The model under review builds one solid part; all positions refer to its coordinate system, in mm. Coordinates: 2 decimals unless noted, no trailing zeros. Order: outer loops, then holes, each group sorted by start corner. A loop starts at its lowest first (then second) coordinate and runs counter-clockwise, first axis right, second up. Notation, with made-up numbers: M 66.5,54.25 L 125.5,54.25 A10 cw 125.5,70.25 Z; hole C 14.25,53 d9. An arc over 180 degrees is marked long. Answer in a Markdown table with one row per item.
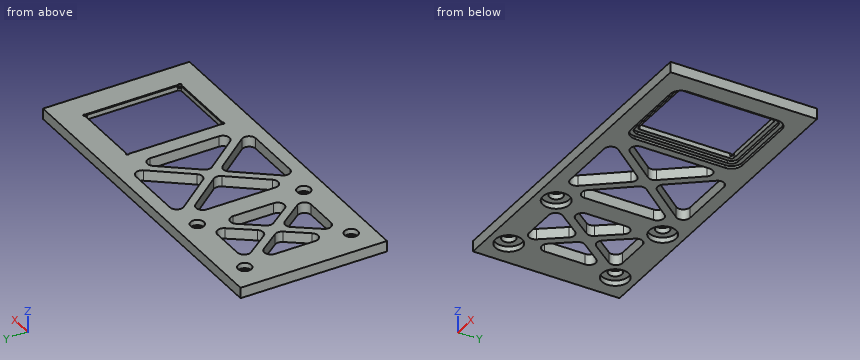
from build123d import *

# Parameters (mm, degrees)
SKETCH1_W           = 125
SKETCH1_H           = 55
SKETCH1_R           = 2.5
SKETCH1_W_2         = 27.05
SKETCH1_H_2         = 35.85
BOSS_EXTRUDE1_DEPTH = 4
SKETCH2_R           = 0.5
CUT_EXTRUDE1_DEPTH  = 1
FILLET1_R           = 1
FILLET2_R           = 1
SKETCH7_W           = 27.45
SKETCH7_H           = 36.25
CUT_EXTRUDE2_DEPTH  = 0.2
CUT_EXTRUDE3_DEPTH  = 2
CUT_EXTRUDE4_DEPTH  = 1
CUT_EXTRUDE5_DEPTH  = 137.623570441
CUT_EXTRUDE6_DEPTH  = 137.623570441
FILLET3_R           = 2.5
SKETCH12_R          = 5
CUT_EXTRUDE7_DEPTH  = 2


with BuildPart() as part:
    # Sketch1 → Boss-Extrude1 (new body)
    with BuildSketch(Plane.XY):
        with Locations((62.5, 27.5)):
            Rectangle(SKETCH1_W, SKETCH1_H)
        with Locations((10, 47.5)):
            Circle(SKETCH1_R, mode=Mode.SUBTRACT)
        with Locations((40, 47.5)):
            Circle(SKETCH1_R, mode=Mode.SUBTRACT)
        with Locations((10, 7.5)):
            Circle(SKETCH1_R, mode=Mode.SUBTRACT)
        with Locations((40, 7.5)):
            Circle(SKETCH1_R, mode=Mode.SUBTRACT)
        with Locations((101.25, 27.5)):
            Rectangle(SKETCH1_W_2, SKETCH1_H_2, mode=Mode.SUBTRACT)
    extrude(amount=BOSS_EXTRUDE1_DEPTH)

    # Sketch2 → Cut-Extrude1 (cut)
    with BuildSketch(Plane.XY.offset(4)):
        with Locations((87.725, 45.425)):
            Circle(SKETCH2_R)
        with Locations((114.775, 45.425)):
            Circle(SKETCH2_R)
        with Locations((87.725, 9.575)):
            Circle(SKETCH2_R)
        with Locations((114.775, 9.575)):
            Circle(SKETCH2_R)
    extrude(amount=-CUT_EXTRUDE1_DEPTH, mode=Mode.SUBTRACT)

    # Fillet1
    # the kernel refuses this fillet: 1 mm, written as the material it adds along each edge
    with BuildSketch(Plane(origin=(114.775, 9.575, 0), x_dir=(-1, 0, 0), z_dir=(0, 0, 1))) as fillet1_piece_1_section:
        with BuildLine():
            CenterArc((FILLET1_R, -FILLET1_R), FILLET1_R, 90, 90)
            Line((0, -FILLET1_R), (0, 0))
            Line((0, 0), (FILLET1_R, 0))
        make_face()
    fillet1_piece_1 = extrude(amount=5.5, mode=Mode.PRIVATE)
    fillet1_piece_1 = split(fillet1_piece_1, bisect_by=Plane(origin=(114.157064257, 9.617383677, 4), z_dir=(0, 0, -1)), keep=Keep.TOP, mode=Mode.PRIVATE)
    fillet1_piece_1 = fillet1_piece_1 - Plane(origin=(114.775, 9.575, 1.5), x_dir=(1, 0, 0), z_dir=(0, 0, 1)) * Cylinder(0.5, 16, mode=Mode.PRIVATE)
    add(fillet1_piece_1)
    with BuildSketch(Plane(origin=(114.775, 9.575, 0), x_dir=(-1, 0, 0), z_dir=(0, 0, 1)), Plane(origin=(87.725, 9.575, 0), x_dir=(0, 1, 0), z_dir=(0, 0, 1)), Plane(origin=(114.775, 45.425, 0), x_dir=(0, -1, 0), z_dir=(0, 0, 1))) as fillet1_piece_2:
        with BuildLine():
            CenterArc((FILLET1_R, -FILLET1_R), FILLET1_R, 90, 90)
            Line((0, -FILLET1_R), (0, 0))
            Line((0, 0), (FILLET1_R, 0))
        make_face()
    extrude(amount=3)
    with BuildSketch(Plane(origin=(87.725, 9.575, 0), x_dir=(0, 1, 0), z_dir=(0, 0, 1))) as fillet1_piece_3_section:
        with BuildLine():
            CenterArc((FILLET1_R, -FILLET1_R), FILLET1_R, 90, 90)
            Line((0, -FILLET1_R), (0, 0))
            Line((0, 0), (FILLET1_R, 0))
        make_face()
    fillet1_piece_3 = extrude(amount=5.5, mode=Mode.PRIVATE)
    fillet1_piece_3 = split(fillet1_piece_3, bisect_by=Plane(origin=(87.767383677, 10.192935743, 4), z_dir=(0, 0, -1)), keep=Keep.TOP, mode=Mode.PRIVATE)
    fillet1_piece_3 = fillet1_piece_3 - Plane(origin=(87.725, 9.575, 1.5), x_dir=(1, 0, 0), z_dir=(0, 0, 1)) * Cylinder(0.5, 15, mode=Mode.PRIVATE)
    add(fillet1_piece_3)
    with BuildSketch(Plane(origin=(114.775, 45.425, 0), x_dir=(0, -1, 0), z_dir=(0, 0, 1))) as fillet1_piece_4_section:
        with BuildLine():
            CenterArc((FILLET1_R, -FILLET1_R), FILLET1_R, 90, 90)
            Line((0, -FILLET1_R), (0, 0))
            Line((0, 0), (FILLET1_R, 0))
        make_face()
    fillet1_piece_4 = extrude(amount=5.5, mode=Mode.PRIVATE)
    fillet1_piece_4 = split(fillet1_piece_4, bisect_by=Plane(origin=(114.732616323, 44.807064257, 4), z_dir=(0, 0, -1)), keep=Keep.TOP, mode=Mode.PRIVATE)
    fillet1_piece_4 = fillet1_piece_4 - Plane(origin=(114.775, 45.425, 1.5), x_dir=(1, 0, 0), z_dir=(0, 0, 1)) * Cylinder(0.5, 15, mode=Mode.PRIVATE)
    add(fillet1_piece_4)
    with BuildSketch(Plane(origin=(87.725, 45.425, 0), x_dir=(0, -1, 0), z_dir=(0, 0, 1))) as fillet1_piece_5_section:
        with BuildLine():
            CenterArc((FILLET1_R, FILLET1_R), FILLET1_R, 180, 90)
            Line((0, FILLET1_R), (0, 0))
            Line((0, 0), (FILLET1_R, 0))
        make_face()
    fillet1_piece_5 = extrude(amount=5.5, mode=Mode.PRIVATE)
    fillet1_piece_5 = split(fillet1_piece_5, bisect_by=Plane(origin=(87.767383677, 44.807064257, 4), z_dir=(0, 0, -1)), keep=Keep.TOP, mode=Mode.PRIVATE)
    fillet1_piece_5 = fillet1_piece_5 - Plane(origin=(87.725, 45.425, 1.5), x_dir=(1, 0, 0), z_dir=(0, 0, 1)) * Cylinder(0.5, 16, mode=Mode.PRIVATE)
    add(fillet1_piece_5)
    with BuildSketch(Plane(origin=(87.725, 45.425, 0), x_dir=(0, -1, 0), z_dir=(0, 0, 1))) as fillet1_piece_6:
        with BuildLine():
            CenterArc((FILLET1_R, FILLET1_R), FILLET1_R, 180, 90)
            Line((0, FILLET1_R), (0, 0))
            Line((0, 0), (FILLET1_R, 0))
        make_face()
    extrude(amount=3)

    # Fillet2
    # the kernel refuses this fillet: 1 mm, written as the material it takes off along each edge
    with BuildSketch(Plane(origin=(114.297140543, 9.722140543, 5.642166577), x_dir=(-0.9745882982080014, -0.22400368076447263, 0), z_dir=(0, 0, -1)), Plane(origin=(87.872140543, 10.052859457, 5.642166577), x_dir=(-0.22400368076451274, 0.9745882982079922, 0), z_dir=(0, 0, -1)), Plane(origin=(114.627859457, 44.947140543, 5.642166577), x_dir=(0.22400368076446278, -0.9745882982080036, 0), z_dir=(0, 0, -1)), Plane(origin=(88.202859457, 45.277859457, 5.642166577), x_dir=(0.974588298207998, 0.22400368076448807, 0), z_dir=(0, 0, -1))) as fillet2_piece_1:
        with BuildLine():
            CenterArc((0.880870312, -0.974588298), FILLET2_R, 102.944297934, 48.189685104)
            Line((0.005119296, -0.491825252), (-0.082455806, -0.443548947))
            ThreePointArc((-0.082455806, -0.443548947), (-0.032777878, -0.246280446), (-0.086551242, -0.050088746))
            Line((-0.086551242, -0.050088746), (0.031782841, 0.094814825))
            ThreePointArc((0.031782841, 0.094814825), (0.519431718, 0.071018782), (0.634466263, 0.09745883))
            Line((0.634466263, 0.09745883), (0.656866631, 0))
        make_face()
    extrude(amount=2.642166577, mode=Mode.SUBTRACT)
    with BuildSketch(Plane(origin=(114.627859457, 10.052859457, 5.642166577), x_dir=(0.22400368076446103, 0.9745882982080041, 0), z_dir=(0, 0, -1)), Plane(origin=(88.202859457, 9.722140543, 5.642166577), x_dir=(0.9745882982080036, -0.22400368076446323, 0), z_dir=(0, 0, -1)), Plane(origin=(114.297140543, 45.277859457, 5.642166577), x_dir=(-0.974588298207998, 0.22400368076448807, 0), z_dir=(0, 0, -1)), Plane(origin=(87.872140543, 44.947140543, 5.642166577), x_dir=(-0.22400368076451097, -0.9745882982079925, 0), z_dir=(0, 0, -1))) as fillet2_piece_2:
        with BuildLine():
            CenterArc((0.880870312, 0.974588298), FILLET2_R, 208.866016962, 48.189685104)
            Line((0.005119296, 0.491825252), (-0.082455806, 0.443548947))
            ThreePointArc((-0.082455806, 0.443548947), (-0.032777878, 0.246280446), (-0.086551242, 0.050088746))
            Line((-0.086551242, 0.050088746), (0.031782841, -0.094814825))
            ThreePointArc((0.031782841, -0.094814825), (0.519431718, -0.071018782), (0.634466263, -0.09745883))
            Line((0.634466263, -0.09745883), (0.656866631, 0))
        make_face()
    extrude(amount=2.642166577, mode=Mode.SUBTRACT)

    # Sketch7 → Cut-Extrude2 (cut)
    with BuildSketch(Plane.XY.offset(4)):
        with Locations((101.25, 27.5)):
            Rectangle(SKETCH7_W, SKETCH7_H)
    extrude(amount=-CUT_EXTRUDE2_DEPTH, mode=Mode.SUBTRACT)

    # Sketch8 → Cut-Extrude3 (cut)
    with BuildSketch(Plane(origin=(0, 0, 0), x_dir=(-1, 0, 0), z_dir=(0, 0, -1))):
        with BuildLine():
            Line((-116.275, 44.425), (-116.275, 10.575))
            ThreePointArc((-116.275, 10.575), (-115.542766953, 8.807233047), (-113.775, 8.075))
            Line((-113.775, 8.075), (-88.725, 8.075))
            ThreePointArc((-88.725, 8.075), (-86.957233047, 8.807233047), (-86.225, 10.575))
            Line((-86.225, 10.575), (-86.225, 44.425))
            ThreePointArc((-86.225, 44.425), (-86.957233047, 46.192766953), (-88.725, 46.925))
            Line((-88.725, 46.925), (-113.775, 46.925))
            ThreePointArc((-113.775, 46.925), (-115.542766953, 46.192766953), (-116.275, 44.425))
        make_face()
    extrude(amount=-CUT_EXTRUDE3_DEPTH, mode=Mode.SUBTRACT)

    # Sketch9 → Cut-Extrude4 (cut)
    with BuildSketch(Plane(origin=(0, 0, 0), x_dir=(-1, 0, 0), z_dir=(0, 0, -1))):
        with BuildLine():
            Line((-117.775, 44.425), (-117.775, 10.575))
            ThreePointArc((-117.775, 10.575), (-116.603427125, 7.746572875), (-113.775, 6.575))
            Line((-113.775, 6.575), (-88.725, 6.575))
            ThreePointArc((-88.725, 6.575), (-85.896572875, 7.746572875), (-84.725, 10.575))
            Line((-84.725, 10.575), (-84.725, 44.425))
            ThreePointArc((-84.725, 44.425), (-85.896572875, 47.253427125), (-88.725, 48.425))
            Line((-88.725, 48.425), (-113.775, 48.425))
            ThreePointArc((-113.775, 48.425), (-116.603427125, 47.253427125), (-117.775, 44.425))
        make_face()
    extrude(amount=-CUT_EXTRUDE4_DEPTH, mode=Mode.SUBTRACT)

    # Sketch10 → Cut-Extrude5 (cut, through all)
    with BuildSketch(Plane(origin=(0, 0, 0), x_dir=(-1, 0, 0), z_dir=(0, 0, -1))):
        Polygon((-38.2, 42.6), (-26.875, 27.5), (-38.2, 12.4), align=None)
        Polygon((-36.325, 45.1), (-13.675, 45.1), (-25, 30), align=None)
        Polygon((-36.325, 9.9), (-25, 25), (-13.675, 9.9), align=None)
        Polygon((-11.8, 42.6), (-23.125, 27.5), (-11.8, 12.4), align=None)
    extrude(amount=-CUT_EXTRUDE5_DEPTH, mode=Mode.SUBTRACT)

    # Sketch11 → Cut-Extrude6 (cut, through all)
    with BuildSketch(Plane(origin=(0, 0, 0), x_dir=(-1, 0, 0), z_dir=(0, 0, -1))):
        Polygon((-81.725, 47.58754115), (-65.777724276, 27.5), (-81.725, 7.41245885), align=None)
        Polygon((-79.809775724, 50), (-47.915224276, 50), (-63.8625, 29.91245885), align=None)
        Polygon((-79.809775724, 5), (-63.8625, 25.08754115), (-47.915224276, 5), align=None)
        Polygon((-46, 47.58754115), (-61.947275724, 27.5), (-46, 7.41245885), align=None)
    extrude(amount=-CUT_EXTRUDE6_DEPTH, mode=Mode.SUBTRACT)

    # Fillet3
    fillet3_edges = [part.edges().sort_by_distance(p)[0] for p in [
        (25, 30, 2),
        (36.325, 45.1, 2),
        (13.675, 45.1, 2),
        (13.675, 9.9, 2),
        (36.325, 9.9, 2),
        (25, 25, 2),
        (11.8, 42.6, 2),
        (11.8, 12.4, 2),
        (23.125, 27.5, 2),
        (38.2, 12.4, 2),
        (38.2, 42.6, 2),
        (26.875, 27.5, 2),
        (63.8625, 29.91245885, 2),
        (79.809775724, 50, 2),
        (47.915224276, 50, 2),
        (47.915224276, 5, 2),
        (79.809775724, 5, 2),
        (63.8625, 25.08754115, 2),
        (46, 47.58754115, 2),
        (46, 7.41245885, 2),
        (61.947275724, 27.5, 2),
        (81.725, 7.41245885, 2),
        (81.725, 47.58754115, 2),
        (65.777724276, 27.5, 2),
    ]]
    fillet(fillet3_edges, radius=FILLET3_R)

    # Sketch12 → Cut-Extrude7 (cut)
    with BuildSketch(Plane(origin=(0, 0, 0), x_dir=(-1, 0, 0), z_dir=(0, 0, -1))):
        with Locations((-40, 47.5)):
            Circle(SKETCH12_R)
        with Locations((-10, 47.5)):
            Circle(SKETCH12_R)
        with Locations((-40, 7.5)):
            Circle(SKETCH12_R)
        with Locations((-10, 7.5)):
            Circle(SKETCH12_R)
    extrude(amount=-CUT_EXTRUDE7_DEPTH, mode=Mode.SUBTRACT)


solid = part.part
(1) Take a section at B-B (x = 10). Write out the cut boundary in (y, z).
Report:
| item | result |
|---|---|
| outline | M 0,0 L 2.5,0 L 2.5,2 L 5,2 L 5,4 L 0,4 Z; M 10,2 L 12.5,2 L 12.5,0 L 42.5,0 L 42.5,2 L 45,2 L 45,4 L 10,4 Z; M 50,2 L 52.5,2 L 52.5,0 L 55,0 L 55,4 L 50,4 Z |
(2) Take a section at A-A (x = 101.5). Write out the cut boundary in (y, z) (3 decimals).
Report:
| item | result |
|---|---|
| outline | M 0,0 L 6.575,0 L 6.575,1 L 8.075,1 L 8.075,2 L 9.575,2 L 9.575,3.8 L 9.375,3.8 L 9.375,4 L 0,4 Z; M 45.425,2 L 46.925,2 L 46.925,1 L 48.425,1 L 48.425,0 L 55,0 L 55,4 L 45.625,4 L 45.625,3.8 L 45.425,3.8 Z |
(3) To check wall thickness, follow line 1 (X direction, y = 47.5, z = 2.7); line 2 (Y direction, x = 40, z = 2.55); line 3 (Y direction, x = 10, z = 1.45). State the ranges of each line that lie inside material, in increasing order. Write a range as [from, to].
Report:
| item | result |
|---|---|
| line 1 | [0, 7.5], [12.5, 37.5], [42.5, 50.59], [77.13, 125] |
| line 2 | [0, 5], [10, 45], [50, 55] |
| line 3 | [0, 2.5], [12.5, 42.5], [52.5, 55] |
(4) Take a section at C-C (x = 69). Write out the cut boundary in (y, z).
Report:
| item | result |
|---|---|
| outline | M 0,0 L 5,0 L 5,4 L 0,4 Z; M 18.62,0 L 23.44,0 L 23.44,4 L 18.62,4 Z; M 31.56,0 L 36.38,0 L 36.38,4 L 31.56,4 Z; M 50,0 L 55,0 L 55,4 L 50,4 Z |
(5) Insertion check: P1, Ø11.5, axis at x = 40, y = 7.5, coming from the -Z side; P2, Ø5, axis at x = 10, y = 45.5, coming from the -Z side. Each pin has a flat end and moves straight along its axis. Give the tip position at first contact, or say it passes through.
Report:
| item | result |
|---|---|
| P1 | z = 0 |
| P2 | z = 2 |
